```python
from build123d import *

# Parameters (mm, degrees)
SKETCH_R     = 2.75
PAD_DEPTH    = 10
SKETCH002_R  = 1.25
HOLE_DEPTH   = 7.501
CHAMFER_SIZE = 1


with BuildPart() as part:
    # Sketch → Pad (new body)
    with BuildSketch(Plane.XY):
        with BuildLine():
            ThreePointArc((-38.000002, 50), (-45.500002, 42.5), (-38.000002, 35))
            Line((-38.000002, 35), (-15, 35))
            ThreePointArc((-7.5, 27.5), (-9.696699, 32.803301), (-15, 35))
            Line((-7.5, 27.5), (-7.5, -7.5))
            Line((-7.5, -7.5), (7.5, -7.5))
            Line((7.5, 27.5), (7.5, -7.5))
            ThreePointArc((15, 35), (9.696699, 32.803301), (7.5, 27.5))
            Line((15, 35), (38.000002, 35))
            ThreePointArc((38.000002, 35), (45.499998, 42.500002), (37.999998, 50))
            Line((-38.000002, 50), (37.999998, 50))
        make_face()
        with Locations((-38.000002, 42.5)):
            Circle(SKETCH_R, mode=Mode.SUBTRACT)
        with Locations((37.999998, 42.5)):
            Circle(SKETCH_R, mode=Mode.SUBTRACT)
        with BuildLine():
            ThreePointArc((-2.75, 0), (0, -2.75), (2.75, 0))
            Line((2.75, 0), (2.75, 5))
            ThreePointArc((2.75, 5), (0, 7.75), (-2.75, 5))
            Line((-2.75, 0), (-2.75, 5))
        make_face(mode=Mode.SUBTRACT)
    extrude(amount=-PAD_DEPTH)

    # Sketch002 → Hole (cut, through all)
    with BuildSketch(Plane.XZ):
        with Locations((0, -5)):
            Circle(SKETCH002_R)
    extrude(amount=HOLE_DEPTH, mode=Mode.SUBTRACT)

    # Chamfer
    chamfer_edges = [part.edges().sort_by_distance(p)[0] for p in [
        (-1.25, -7.5, -5),
    ]]
    chamfer(chamfer_edges, length=CHAMFER_SIZE)


solid = part.part
```
The model under review builds one solid part; all positions refer to its coordinate system, in mm. A direction names the side the tool comes from. Round coordinates to 2 decimals unless told otherwise and drop trailing zeros. Loops run counter-clockwise (first coordinate to the right, second up) from the corner with the lowest first, then second, coordinate; pieces in that order, holes last. Notation, with made-up numbers: (66.25, 27) -> (112.25, 27) arc R19 ccw to (112.25, 58) -> close; hole circle Ø3 at (14.25, 29). An arc over 180 degrees is marked (long way). Answer in a Markdown table with one row per item.
1) For pin 1 Ø2 at (y, z) = (40.5, -3.5) entering from +X; pin 2 Ø4 at (x, y) = (10.5, 11.5) entering from -Z; pin 3 Ø1 at (x, z) = (20.5, -7.5) entering from -Y; pin 4 Ø5.5 at (y, z) = (3.5, -5) entering from -X, all flat-tipped, find the tip position at first contact; note any pin that passes through.
Taken from the geometry:
| item | result |
|---|---|
| pin 1 | stops at x = 45.43 |
| pin 2 | passes through |
| pin 3 | stops at y = 35 |
| pin 4 | stops at x = -7.5 |
2) Wall thickness on line 1 along Z through (x, y) = (0, -4.2); line 2 along X through (y, z) = (-5.6, -5); line 3 along Y through (x, z) = (-21.5, -4.5): over which ranges is each line inside the solid? List them lowest first.
Taken from the geometry:
| item | result |
|---|---|
| line 1 | z = -10 to -6.25, -3.75 to 0 |
| line 2 | x = -7.5 to -1.25, 1.25 to 7.5 |
| line 3 | y = 35 to 50 |
3) Consider section C-C, the plane z = -1.5. Write out the cut boundary in (x, y).
Taken from the geometry:
| item | result |
|---|---|
| outline | (-38, 35) -> (-15, 35) arc R7.5 cw to (-7.5, 27.5) -> (-7.5, -7.5) -> (7.5, -7.5) -> (7.5, 27.5) arc R7.5 cw to (15, 35) -> (38, 35) arc R7.5 ccw to (38, 50) -> (-38, 50) arc R7.5 ccw to start; hole circle Ø5.5 at (-38, 42.5); hole (-2.75, 0) arc R2.75 ccw to (2.75, 0) -> (2.75, 5) arc R2.75 ccw to (-2.75, 5) -> close; hole circle Ø5.5 at (38, 42.5) |
4) Draft analysis for pull direction X (two halves, no side actions). For faces 6 (the flat face through (7.5, 10, -5)), 7 (the cylindrical face through (-36.52, 44.82, -4.93)), 8 (the cylindrical face through (-9.639, 32.745, -4.93)), 9 (the flat face through (-1, 50, -5)), state which applies: pulls with the +X half, pulls with the -X half, needs draft (parallel to the pull), parting line crosses it, or undercut.
Taken from the geometry:
| item | result |
|---|---|
| face 6 | pulls with the +X half |
| face 7 | undercut |
| face 8 | pulls with the -X half |
| face 9 | needs draft |
5) Consider section B-B, the plane y = 42.5. Write out the cut boundary in (x, z), plus the area to 3 significant figures.
Taken from the geometry:
| item | result |
|---|---|
| outline | (-45.5, -10) -> (-40.75, -10) -> (-40.75, 0) -> (-45.5, 0) -> close; (-35.25, -10) -> (35.25, -10) -> (35.25, 0) -> (-35.25, 0) -> close; (40.75, -10) -> (45.5, -10) -> (45.5, 0) -> (40.75, 0) -> close |
| area | 800 mm² |
6) Consider section D-D, the plane y = 4. Write out the cut boundary in (x, z), plus the area to 3 significant figures.
Taken from the geometry:
| item | result |
|---|---|
| outline | (-7.5, -10) -> (-2.75, -10) -> (-2.75, 0) -> (-7.5, 0) -> close; (2.75, -10) -> (7.5, -10) -> (7.5, 0) -> (2.75, 0) -> close |
| area | 95.0 mm² |
7) Tool access review of faces 1 (the flat face through (26, 35, -5)), 2 (the cylindrical face through (-1.25, -4.45, -4.95)), 3 (the flat face through (-2.75, 2, -5)), 4 (the flat face through (-2, -7.5, -3)), 5 (the flat face through (-7.5, 10, -5)): name each direction out of +Z, -Z, +X, -X, +Y, -Y from which nothing blocks a thin tool from reaching the whole face with its end or side.
Taken from the geometry:
| item | result |
|---|---|
| face 1 | +Z, -Z, +X, -Y |
| face 2 | -Y |
| face 3 | +Z, -Z |
| face 4 | +Z, -Z, +X, -X, -Y |
| face 5 | +Z, -Z, -X, -Y |
8) Consider section A-A, the plane x = 0. Write out the cut boundary in (y, z), plus the area to 3 significant figures.
Taken from the geometry:
| item | result |
|---|---|
| outline | (-7.5, -10) -> (-2.75, -10) -> (-2.75, -6.25) -> (-6.5, -6.25) -> (-7.5, -7.25) -> close; (-7.5, -2.75) -> (-6.5, -3.75) -> (-2.75, -3.75) -> (-2.75, 0) -> (-7.5, 0) -> close; (7.75, -10) -> (50, -10) -> (50, 0) -> (7.75, 0) -> close |
| area | 457 mm² |
